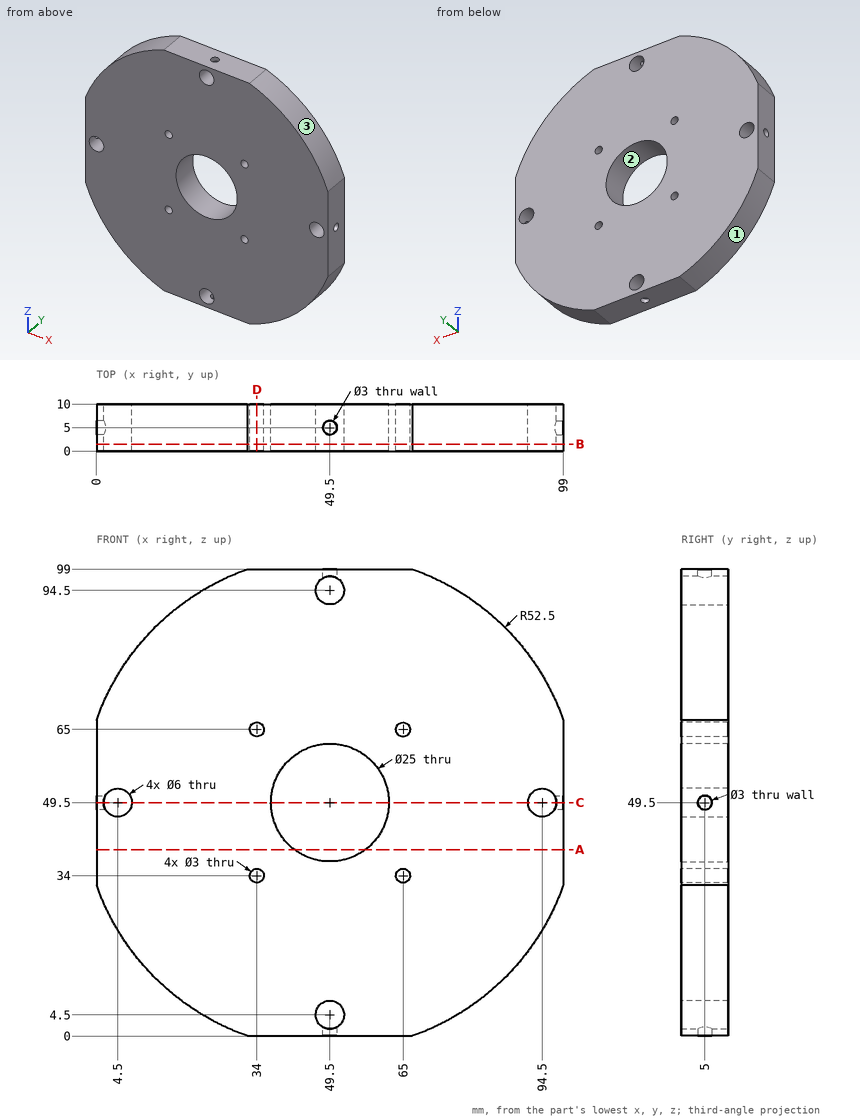
Drawing for the job (mm, zero at the part's lowest x, y, z). Coordinates: 2 decimals unless noted, no trailing zeros. Order: outer loops, then holes, each group sorted by start corner. A loop starts at its lowest first (then second) coordinate and runs counter-clockwise, first axis right, second up.
Item 1: Drill centre lines: L1, parallel to X at y = 3.25, z = 34; L2, parallel to X at y = 5.75, z = 49.5; L3, parallel to Y at x = 0.9, z = 49.5. Where is each one in solid material? Low to high.
Check sheet entries:
L1: x = 0 to 32.5, 35.5 to 63.5, 66.5 to 99
L2: x = 7.5 to 37, 62 to 91.5
L3: y = 0 to 3.5, 6.5 to 10
Item 2: Band-saw the part on D-D on x = 34. List the corners of the cut face in (y, z).
Check sheet entries:
outline: (0, 0) - (10, 0) - (10, 32.5) - (0, 32.5) - close; (0, 35.5) - (10, 35.5) - (10, 63.5) - (0, 63.5) - close; (0, 66.5) - (10, 66.5) - (10, 99) - (0, 99) - close
Item 3: Band-saw the part on B-B on y = 1.5. Give the number of separate pieces and of enclosed holes in the cut face, plus the area to 3 significant figures.
Check sheet entries:
separate pieces: 1
enclosed holes: 9
area: 7,750 mm2
Item 4: Pin check, flat tips, straight feed: pin 1 Ø6 at (x, y) = (11.5, 5) entering from +Z; pin 2 Ø1.8 at (x, y) = (49.5, 5) entering from +Z; pin 3 Ø6 at (y, z) = (5.5, 85.5) entering from -X. Stop position of each tip, or through.
Check sheet entries:
pin 1: stops at z = 88.63
pin 2: stops at z = 91.64
pin 3: stops at x = 8.67
Item 5: Two-plate mould, pull along X, no slides. Class the marked faces 1, 2 and 3: +X half, -X half, draft (parallel to the pull), parting line (faces both ways), or undercut.
Check sheet entries:
face 1: -X half
face 2: undercut
face 3: +X half
Item 6: Band-saw the part on A-A on z = 39.5. List the corners of the cut face in (x, y).
Check sheet entries:
outline: (0, 0) - (42, 0) - (42, 10) - (0, 10) - close; (57, 0) - (99, 0) - (99, 10) - (57, 10) - close
Item 7: Band-saw the part on C-C on z = 49.5. List the corners of the cut face in (x, y).
Check sheet entries:
outline: (0, 0) - (1.5, 0) - (1.5, 3.5) - (0, 3.5) - close; (0, 6.5) - (1.5, 6.5) - (1.5, 10) - (0, 10) - close; (7.5, 0) - (37, 0) - (37, 10) - (7.5, 10) - close; (62, 0) - (91.5, 0) - (91.5, 10) - (62, 10) - close; (97.5, 0) - (99, 0) - (99, 3.5) - (97.5, 3.5) - close; (97.5, 6.5) - (99, 6.5) - (99, 10) - (97.5, 10) - close
